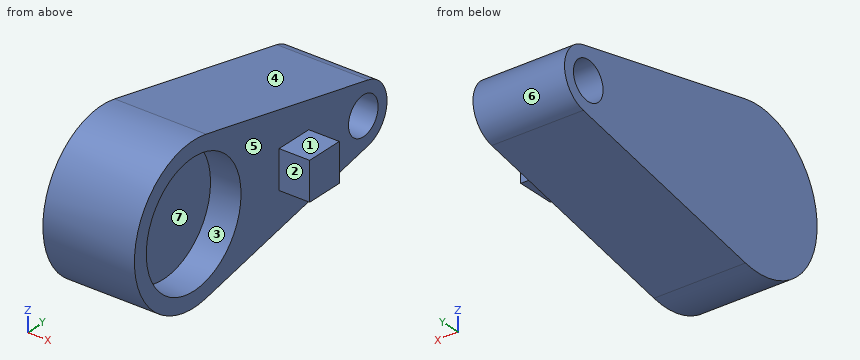
```python
from build123d import *

# Parameters (mm, degrees)
F1_DEPTH = 76.2
F2_R     = 50.8
F3_DEPTH = 25.4
F4_W     = 31.75
F4_H     = 31.75
F5_DEPTH = 25.4
F6_R     = 15.875
F7_DEPTH = 76.2


with BuildPart() as f1:
    # F0 (on Right) → F1 (new body)
    with BuildSketch(Plane.YZ):
        with BuildLine():
            ThreePointArc((13.3050971344, -62.0904532939), (49.3817965856, -39.9210241099), (63.5, 0))
            ThreePointArc((63.5, 0), (49.3817965856, 39.9210241099), (13.3050971344, 62.0904532939))
            ThreePointArc((13.3050971344, 62.0904532939), (-63.5, 0), (13.3050971344, -62.0904532939))
        make_face()
        with BuildLine():
            ThreePointArc((13.3050971344, 62.0904532939), (49.3817965856, 39.9210241099), (63.5, 0))
            ThreePointArc((63.5, 0), (49.3817965856, -39.9210241099), (13.3050971344, -62.0904532939))
            Line((13.3050971344, -62.0904532939), (187.1583663574, -24.8361813176))
            ThreePointArc((187.1583663574, -24.8361813176), (156.4363275036, 0), (187.1583663574, 24.8361813176))
            Line((187.1583663574, 24.8361813176), (13.3050971344, 62.0904532939))
        make_face()
        with BuildLine():
            ThreePointArc((207.2363275036, 0), (201.5890461378, 15.968409644), (187.1583663574, 24.8361813176))
            ThreePointArc((187.1583663574, 24.8361813176), (156.4363275036, 0), (187.1583663574, -24.8361813176))
            ThreePointArc((187.1583663574, -24.8361813176), (201.5890461378, -15.968409644), (207.2363275036, 0))
        make_face()
    extrude(amount=F1_DEPTH)

    # F2 (on face) → F3 (cut)
    with BuildSketch(Plane.YZ.offset(76.2)):
        Circle(F2_R)
    extrude(amount=-F3_DEPTH, mode=Mode.SUBTRACT)

    # F4 (on face) → F5 (join)
    with BuildSketch(Plane.YZ.offset(76.2)):
        with Locations((107.4921913939, 0)):
            Rectangle(F4_W, F4_H)
    extrude(amount=F5_DEPTH)

    # F6 (on face) → F7 (cut, through all)
    with BuildSketch(Plane.YZ.offset(76.2)):
        with Locations((181.8363275036, 0)):
            Circle(F6_R)
    extrude(amount=-F7_DEPTH, mode=Mode.SUBTRACT)


solid = f1.part
```
Check sheet for the modelled part. Datum: model origin and axes. Units: mm. Face numbers are marked on the shaded views. A direction names the side the tool comes from. Round coordinates to 2 decimals unless told otherwise and drop trailing zeros. Loops run counter-clockwise (first coordinate to the right, second up) from the corner with the lowest first, then second, coordinate; pieces in that order, holes last. Notation, with made-up numbers: (7.25, -13) - (57.25, -13) arc R15 cw to (57.25, 14) - close; hole circle Ø2 at (-2, 56.25). An arc over 180 degrees is marked (long way). Answer as a JSON object with one key per item and string values. Group by question number.
Q1. Sectioned sample at A-A, the plane z = 0. Enter the section's corners in (x, y), plus the area to 3 significant figures.
Q2. Sectioned sample at C-C, the plane y = 0. Enter the section's corners in (x, z).
Q3. Sectioned sample at D-D, the plane z = -42. Enter the section's corners in (x, y).
Q4. Mould release check, pull along Y, two halves, no side actions. Record for the marked faces 5, 6 and 7: released by +Y, released by -Y, zero draft, split by the parting line, or undercut.
Q5. Gauge pin test, flat ends, axial feed: P1, Ø6, axis at x = 30.5, y = 48, coming from the +Z side; P2, Ø6, axis at x = 13.5, z = -47, coming from the -Y side; P3, Ø1, axis at x = 41, y = -12, coming from the +Z side. Record the tip position at first contact, or that the pin passes through.
Q6. Scan lines: line 1 along Z through (x, y) = (59, 0); line 2 along X through (y, z) = (-41.5, -15.5); line 3 along X through (y, z) = (154.5, 15). Record each from-to range of solid material in increasing order. Write a range as [from, to].
Q7. Sectioned sample at B-B, the plane x = 11. Enter the section's corners in (y, z) (3 decimals), plus the area to 3 significant figures.
Q8. Set-up check for the marked faces 1, 2, 3 and 4: record each of +Z, -Z, +X, -X, +Y, -Y from which the full face is reachable in a straight line by a thin tool's end or side.
Solution:
{
 "1": {"outline": "(0, -63.5) - (76.2, -63.5) - (76.2, -50.8) - (50.8, -50.8) - (50.8, 50.8) - (76.2, 50.8) - (76.2, 91.62) - (101.6, 91.62) - (101.6, 123.37) - (76.2, 123.37) - (76.2, 165.96) - (0, 165.96) - close; (0, 197.71) - (76.2, 197.71) - (76.2, 207.24) - (0, 207.24) - close", "area": "16,400 mm²"},
 "2": {"outline": "(0, -63.5) - (76.2, -63.5) - (76.2, -50.8) - (50.8, -50.8) - (50.8, 50.8) - (76.2, 50.8) - (76.2, 63.5) - (0, 63.5) - close"},
 "3": {"outline": "(0, -47.63) - (76.2, -47.63) - (76.2, -28.58) - (50.8, -28.58) - (50.8, 28.58) - (76.2, 28.58) - (76.2, 107.06) - (0, 107.06) - close"},
 "4": {"face 5": "zero draft", "face 6": "released by +Y", "face 7": "undercut"},
 "5": {"P1": "stops at z = 55.3", "P2": "stops at y = -45.78", "P3": "stops at z = 62.45"},
 "6": {"line 1": "z = [-63.5, -50.8], [50.8, 63.5]", "line 2": "x = [0, 50.8]", "line 3": "x = [0, 76.2]"},
 "7": {"outline": "(13.305, -62.09) - (187.158, -24.836) arc R25.4 ccw to (187.158, 24.836) - (13.305, 62.09) arc R63.5 ccw (long way) to start; hole circle Ø31.75 at (181.836, 0)", "area": "23,100 mm²"},
 "8": {"face 1": "+Z, +X, +Y, -Y", "face 2": "+Z, -Z, +X, -Y", "face 3": "+X", "face 4": "+Z, +X, -X, +Y"}
}
